Build history of the part. All positions in model axes, mm. Face numbers are marked on the shaded views. A direction names the side the tool comes from. Coordinates: 2 decimals unless noted, no trailing zeros. Order: outer loops, then holes, each group sorted by start corner. A loop starts at its lowest first (then second) coordinate and runs counter-clockwise, first axis right, second up. Notation, with made-up numbers: (-11.75, -25) -> (11.25, -25) arc R13 ccw to (11.25, -2) -> close; hole circle Ø6 at (1.25, 83.25). An arc over 180 degrees is marked (long way). Write each question's results on one line, items separated by ' | '.
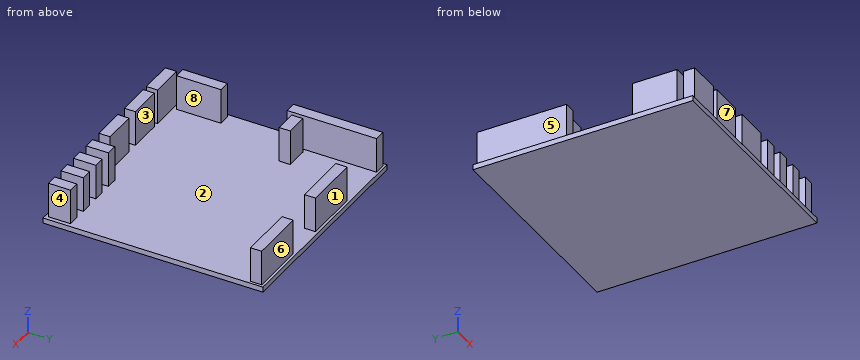
from build123d import *

# Parameters (mm, degrees)
CROQUIS1_W              = 50
CROQUIS1_H              = 50
SALIENTE_EXTRUIR1_DEPTH = 1.2
CROQUIS2_W              = 12.7
CROQUIS2_H              = 2.54
CROQUIS2_W_2            = 2.54
CROQUIS2_H_2            = 20.32
CROQUIS2_W_3            = 5.08
CROQUIS2_H_3            = 10.16
CROQUIS2_W_4            = 7.62
CROQUIS2_H_4            = 5.08
SALIENTE_EXTRUIR2_DEPTH = 8


with BuildPart() as part:
    # Croquis1 → Saliente-Extruir1 (new body)
    with BuildSketch(Plane.XY):
        with Locations((25, 25)):
            Rectangle(CROQUIS1_W, CROQUIS1_H)
    extrude(amount=SALIENTE_EXTRUIR1_DEPTH)

    # Croquis2 → Saliente-Extruir2 (add)
    with BuildSketch(Plane.XY.offset(1.2)):
        with Locations((43.05, 48.13)):
            Rectangle(CROQUIS2_W, CROQUIS2_H)
        with Locations((21.35, 48.13)):
            Rectangle(CROQUIS2_W, CROQUIS2_H)
        with Locations((2.07, 39.34)):
            Rectangle(CROQUIS2_W_2, CROQUIS2_H_2)
        with Locations((6.84, 32.03)):
            Rectangle(CROQUIS2_W_3, CROQUIS2_H)
        with Locations((2.07, 9.08)):
            Rectangle(CROQUIS2_W_2, CROQUIS2_H_3)
        with Locations((5.81, 1.97)):
            Rectangle(CROQUIS2_W_4, CROQUIS2_H)
        with Locations((14.69, 1.97)):
            Rectangle(CROQUIS2_W_4, CROQUIS2_H)
        with Locations((24.91, 1.97)):
            Rectangle(CROQUIS2_W_4, CROQUIS2_H)
        with Locations((32.59, 3.24)):
            Rectangle(CROQUIS2_W_2, CROQUIS2_H_4)
        with Locations((37.67, 3.24)):
            Rectangle(CROQUIS2_W_2, CROQUIS2_H_4)
        with Locations((42.75, 3.24)):
            Rectangle(CROQUIS2_W_2, CROQUIS2_H_4)
        with Locations((47.83, 3.24)):
            Rectangle(CROQUIS2_W_2, CROQUIS2_H_4)
    extrude(amount=SALIENTE_EXTRUIR2_DEPTH)


solid = part.part
Item 1: Pin check, flat tips, straight feed: pin 1 (1 mm diameter, centred on x = 14.5, y = 26, fed in from -Z); pin 2 (1.3 mm diameter, centred on x = 48, z = 6.5, fed in from -Y); pin 3 (1.3 mm diameter, centred on y = 48.5, z = 3.5, fed in from +X); pin 4 (4 mm diameter, centred on x = 19, z = 3.5, fed in from +Y). Stop position of each tip, or through.
Answer:
pin 1: stops at z = 0 | pin 2: stops at y = 0.7 | pin 3: stops at x = 49.4 | pin 4: stops at y = 49.4
Item 2: Slice it at C-C, the plane y = 25. List the corners of the cut face in (x, z).
Answer:
outline: (0, 0) -> (50, 0) -> (50, 1.2) -> (0, 1.2) -> close
Item 3: Slice it at A-A, the plane y = 9. List the corners of the cut face in (x, z), and give its area (3 significant figures).
Answer:
outline: (0, 0) -> (50, 0) -> (50, 1.2) -> (3.34, 1.2) -> (3.34, 9.2) -> (0.8, 9.2) -> (0.8, 1.2) -> (0, 1.2) -> close | area: 80.3 mm^2
Item 4: Drill centre lines: line 1 (Y direction, x = 2.5, z = 3.25); line 2 (X direction, y = 32, z = 7); line 3 (Y direction, x = 6, z = 7.25). Where is each one in solid material? Low to high. Write a range as from..to.
Answer:
line 1: y = 0.7..3.24, 4..14.16, 29.18..49.5 | line 2: x = 0.8..3.34, 4.3..9.38 | line 3: y = 0.7..3.24, 30.76..33.3
Item 5: Slice it at B-B, the plane z = 7. State how many separate pieces and enclosed holes the cut face has, and give its area (3 significant figures).
Answer:
separate pieces: 12 | enclosed holes: 0 | area: 265 mm^2
Item 6: Pull direction Y, two halves, no side cores. Call the marked faces 1, 2, 3 and 4: released by +Y, released by -Y, zero draft, split by the parting line, or undercut.
Answer:
face 1: released by +Y | face 2: undercut | face 3: undercut | face 4: zero draft
Item 7: Tool access for the marked faces 5, 6, 7 and 8: list every direction of +Z, -Z, +X, -X, +Y, -Y with a clear straight run to the whole face (end or side of a thin tool).
Answer:
face 5: +Z, -X, +Y, -Y | face 6: +Z, +X, +Y | face 7: +Z, +X, -X, -Y | face 8: +Z, +Y
